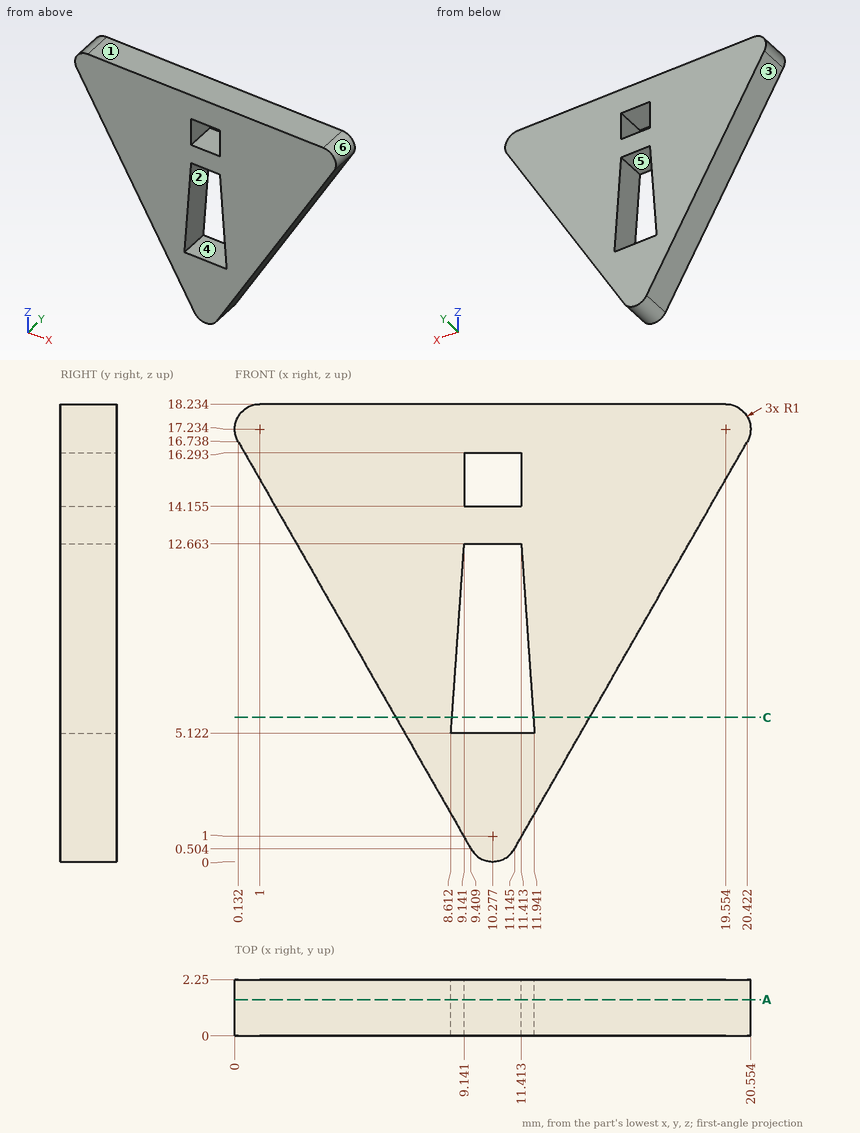
Answer from the drawing. Dimensions are ordinates in mm from the lowest x, y and z of the part. A direction names the side the tool comes from. Coordinates: 2 decimals unless noted, no trailing zeros. Loops run counter-clockwise (first coordinate to the right, second up) from the corner with the lowest first, then second, coordinate; pieces in that order, holes last. Notation, with made-up numbers: (3, 16.5) -> (9, 16.5) arc R28 cw to (9, 36.5) -> close; hole circle Ø6 at (-11, 87). An arc over 180 degrees is marked (long way). Answer in a Markdown table with one row per item.
Item 1: For a pull along Z with two mould halves and no side action, classify the marked faces 3, 4, 5 and 6 as released by +Z, released by -Z, zero draft, split by the parting line, or undercut.
Returned:
| item | result |
|---|---|
| face 3 | released by -Z |
| face 4 | undercut |
| face 5 | undercut |
| face 6 | split by the parting line |
Item 2: For the marked faces 1 and 2, determine the directions among +Z, -Z, +X, -X, +Y, -Y from which every point of the face is accessible in a straight line to the end or side of a thin tool.
Returned:
| item | result |
|---|---|
| face 1 | +Z, +X, -X, +Y, -Y |
| face 2 | +Y, -Y |
Item 3: A cutting plane is placed at C-C on z = 5.75. Determine the outline of the cut face in (x, y), plus the area to 3 significant figures.
Returned:
| item | result |
|---|---|
| outline | (6.41, 0) -> (8.66, 0) -> (8.66, 2.25) -> (6.41, 2.25) -> close; (11.9, 0) -> (14.14, 0) -> (14.14, 2.25) -> (11.9, 2.25) -> close |
| area | 10.1 mm^2 |
Item 4: Straight lines are drawn through the part: line 1 along Z through (x, y) = (11, 0.6) (1 decimal); line 2 along X through (y, z) = (1, 10.25) (1 decimal); line 3 along X through (y, z) = (1.6, 9.5) (1 decimal). For each, find the intervals that lie inside material, in ascending order. Write a range as [from, to].
Returned:
| item | result |
|---|---|
| line 1 | z = [0.3, 5.1], [12.7, 14.2], [16.3, 18.2] |
| line 2 | x = [3.8, 9], [11.6, 16.7] |
| line 3 | x = [4.3, 8.9], [11.6, 16.3] |
Item 5: A cutting plane is placed at A-A on y = 1.45. Determine the outline of the cut face in (x, z) (1 decimal), plus the area to 3 significant figures.
Returned:
| item | result |
|---|---|
| outline | (0.1, 16.7) -> (9.4, 0.5) arc R1 ccw to (11.1, 0.5) -> (20.4, 16.7) arc R1 ccw to (19.6, 18.2) -> (1, 18.2) arc R1 ccw to start; hole (8.6, 5.1) -> (11.9, 5.1) -> (11.4, 12.7) -> (9.1, 12.7) -> close; hole (9.1, 14.2) -> (11.4, 14.2) -> (11.4, 16.3) -> (9.1, 16.3) -> close |
| area | 184 mm^2 |
